Job drawing, mm, ordinate dimensions from the low corner. One solid piece. Coordinates: 2 decimals unless noted, no trailing zeros. Write each loop counter-clockwise with the first axis right and the second up, starting at its lowest first coordinate (ties: lowest second). Pieces come first, ordered by that corner, then holes. Notation, with made-up numbers: (-12.5, 4) -> (46.5, 4) arc R19 ccw to (46.5, 23) -> close; hole circle Ø8 at (27.5, -28.75). An arc over 180 degrees is marked (long way). Answer as a JSON object with one key per item and string values. Group by question number.
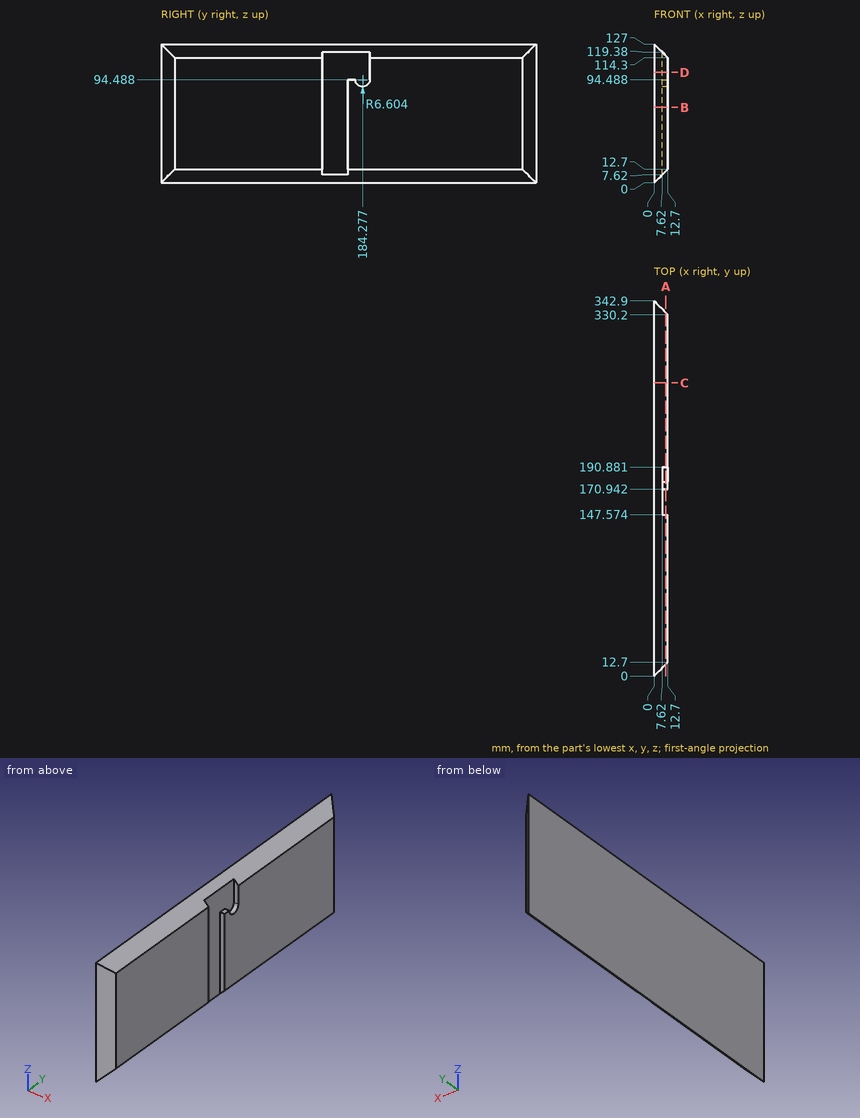
(1) Cut at D-D on z = 101. List the corners of the cut face in (x, y), plus the area to 3 significant figures.
(2) Cut at B-B on z = 69. List the corners of the cut face in (x, y).
(3) Wall check: probe 1 along Y at (x, z) = (8.25, 22); probe 2 along Y at (x, z) = (7.75, 19); probe 3 along Z at (x, y) = (7, 316). Give the ranges that are in metal, low to high.
(4) Cut at C-C on y = 268. List the corners of the cut face in (x, z), plus the area to 3 significant figures.
(5) Cut at A-A on x = 10.75. List the corners of the cut face in (y, z), plus the area to 3 significant figures.
(6) Pin check, flat tips, straight feed: pin 1 (2 mm diameter, centred on x = 8.5, z = 66.5, fed in from +Y); pin 2 (4 mm diameter, centred on x = 11.5, y = 175.5, fed in from +Z); pin 3 (1.5 mm diameter, centred on x = 11, z = 81.5, fed in from +Y). Stop position of each tip, or through.
Results found:
{
 "1": {"outline": "(0, 0) -> (12.7, 12.7) -> (12.7, 147.57) -> (7.62, 147.57) -> (7.62, 190.88) -> (12.7, 190.88) -> (12.7, 330.2) -> (0, 342.9) -> close", "area": "3,970 mm²"},
 "2": {"outline": "(0, 0) -> (12.7, 12.7) -> (12.7, 147.57) -> (7.62, 147.57) -> (7.62, 170.94) -> (12.7, 170.94) -> (12.7, 330.2) -> (0, 342.9) -> close"},
 "3": {"probe 1": "y = 8.25 to 147.57, 170.94 to 334.65", "probe 2": "y = 7.75 to 147.57, 170.94 to 335.15", "probe 3": "z = 7 to 120"},
 "4": {"outline": "(0, 0) -> (12.7, 12.7) -> (12.7, 114.3) -> (0, 127) -> close", "area": "1,450 mm²"},
 "5": {"outline": "(10.75, 10.75) -> (147.57, 10.75) -> (147.57, 116.25) -> (10.75, 116.25) -> close; (170.94, 10.75) -> (332.15, 10.75) -> (332.15, 116.25) -> (190.88, 116.25) -> (190.88, 94.49) arc R6.6 cw to (177.67, 94.49) -> (170.94, 94.49) -> close", "area": "30,900 mm²"},
 "6": {"pin 1": "stops at y = 335.4", "pin 2": "stops at z = 94.49", "pin 3": "stops at y = 332.65"}
}
